Autodesk Inventor part; units mm, degrees
ref_plane "YZ Plane" through (0, 0, 0) normal (1, 0, 0) x (0, 1, 0)
ref_plane "XZ Plane" through (0, 0, 0) normal (0, 1, 0) x (-1, 0, 0)
ref_plane "XY Plane" through (0, 0, 0) normal (0, 0, 1) x (1, 0, 0)
sketch "Szkic1" plane through (0, 0, 0) normal (0, 1, 0) x (-1, 0, 0)
  line L0 (-15, 0) -> (-85, 0)
  line L1 (-100, -15) -> (-100, -100)
  line L2 (-100, -100) -> (0, -100)
  line L3 (0, -100) -> (0, -15)
  arc A0 (0, -15) -> (-15, 0) centre (-15, -15) ccw
  arc A1 (-85, 0) -> (-100, -15) centre (-85, -15) ccw
  point P0 (0, 0)
  point P1 (-100, 0)
  dimension "d0" = 100
  dimension "d1" = 100
  dimension "d2" = 15
extrude "Wyciągnięcie proste1" add sketch "Szkic1" along normal blind 10
sketch "Szkic2" plane through (0, 10, 0) normal (0, 1, 0) x (1, 0, 0)
  line L0 (0, 100) -> (100, 100)
  line L1 (100, 100) -> (100, 50)
  line L2 (100, 50) -> (0, 50)
  line L3 (0, 50) -> (0, 100)
  point P0 (0, 0)
  dimension "d5" = 100
  dimension "d6" = 50
extrude "Wyciągnięcie proste2" add sketch "Szkic2" along normal blind 20
sketch "Szkic3" plane through (0, 10, 0) normal (0, 1, 0) x (1, 0, 0)
  arc A0 (0, 15) -> (15, 0) centre (15, 15) ccw
  arc A1 (85, 0) -> (100, 15) centre (85, 15) ccw
  point P0 (0, 0)
hole "Otwór1" at (15, 10, -15) at (85, 10, -15) direction (0, -1, 0) diameter 16 end through all
mirror "Odbij1" about plane through (50, 30, -75) normal (0, 1, 0) of "Wyciągnięcie proste1", "Otwór1", "Wyciągnięcie proste2"
sketch "Szkic4" plane through (100, 0, -100) normal (0, 0, -1) x (-1, 0, 0)
  circle A0 centre (-40, 19) radius 19
  line L0 (15, 0) -> (0, 0)
  line L1 (0, 0) -> (-40, 0)
  line L2 (-40, 38) -> (0, 38)
  line L3 (0, 10) -> (0, 50)
  line L4 (0, 0) -> (0, 38)
  point P0 (100, 0)
  dimension "d16" = 38
  dimension "d17" = 40
extrude "Wyciągnięcie proste3" add sketch "Szkic4" against normal blind 12
sketch "Szkic5" plane through (100, 60, -100) normal (0, 0, -1) x (-1, 0, 0)
  arc A0 (-40, -22) -> (-40, -60) centre (-40, -41) ccw
  circle A1 centre (-40, -41) radius 19
  point P0 (100, -60)
  point P1 (-40, -22)
  dimension "d20" = 38
extrude "Wyciągnięcie proste4" add sketch "Szkic5" along normal blind 28
sketch "Szkic6" plane through (140, 19, -128) normal (0, 0, -1) x (-1, 0, 0)
  point P0 (140, -19)
  point P1 (0, 0)
hole "Otwór2" at (140, 19, -128) direction (0, 0, 1) diameter 24 end through all
fillet "Zaokrąglenie1" radius 6 1 edges at (100, 19, -88)
sketch "Szkic7" plane through (0, 0, -100) normal (-1, 0, 0) x (0, 0, 1)
  circle A0 centre (19, 100) radius 19
  line L0 (0, 0) -> (0, 60)
  line L1 (0, 60) -> (0, 100)
  line L2 (38, 100) -> (38, 60)
  line L3 (0, 60) -> (85, 60)
  point P0 (100, 0)
  dimension "d31" = 38
  dimension "d32" = 40
extrude "Wyciągnięcie proste5" add sketch "Szkic7" against normal blind 12
sketch "Szkic8" plane through (0, 0, -100) normal (-1, 0, 0) x (0, 0, 1)
  arc A0 (38, 100) -> (0, 100) centre (19, 100) ccw
  circle A1 centre (19, 100) radius 19
  point P0 (100, 0)
  dimension "d35" = 38
extrude "Wyciągnięcie proste6" add sketch "Szkic8" along normal blind 38
sketch "Szkic9" plane through (-38, 100, -81) normal (-1, 0, 0) x (0, 0, 1)
  point P0 (81, -100)
  point P1 (0, 0)
hole "Otwór3" at (-38, 100, -81) direction (1, 0, 0) diameter 22 end through all
fillet "Zaokrąglenie2" radius 6 1 edges at (12, 60, -81)
The listing builds one solid part. Answer for the finished solid, in the listing's coordinates (mm). A direction names the side the tool comes from. Round coordinates to 2 decimals unless told otherwise and drop trailing zeros. Loops run counter-clockwise (first coordinate to the right, second up) from the corner with the lowest first, then second, coordinate; pieces in that order, holes last.
Q1. Section B-B, the plane x = 3 is taken. Determine the outline of the cut face in (y, z).
Q2. Section C-C, the plane z = -26 is taken. Determine the outline of the cut face in (x, y), then the cut area to 3 significant figures.
Q3. Find the intervals of material crossed by line 1 (X direction, y = 6.75, z = -15); line 2 (Z direction, x = 15, y = 7.25); line 3 (Y direction, x = 22, z = -35), in increasing order.
Q4. For a pull along Z with two mould halves and no side action, classify faces 1 (the face through (140.3, 6.6, -128)), 2 (the face through (15, 5, -23)), 3 (the face through (95.72, 4.93, -4.51)) as released by +Z, released by -Z, zero draft, split by the parting line, or undercut.
Q5. Given pin 1 Ø14.5 at (x, y) = (10, 70.5) entering from +Z; pin 2 Ø14.5 at (x, z) = (85, -15) entering from -Y; pin 3 Ø8 at (y, z) = (68, -76.5) entering from +X; pin 4 Ø6 at (x, y) = (116.5, 37.5) entering from -Z, each flat-ended and moving along its own axis, determine where each tip first touches the part or whether it passes through.
Q6. Section A-A, the plane y = 19 is taken. Determine the outline of the cut face in (x, z).
Q7. Section D-D, the plane z = -94.5 is taken. Determine the outline of the cut face in (x, y), then the cut area to 3 significant figures.
Q8. Which of the six approach directions +Z, -Z, +X, -X, +Y, -Y give full straight-line access (tool end or side, diameter ignored) to faces 4 (the face through (127, 19, -88)), 5 (the face through (49, 60, -49)), 6 (the face through (120, 38, -93)), 7 (the face through (-12.65, 118.548, -85.119))?
Completed:
1. outline: (0, -100) - (100, -100) arc R19 ccw to (100, -62) - (60, -62) - (60, -6) - (50, -6) - (50, -50) - (10, -50) - (10, -6) - (0, -6) - close; hole circle Ø22 at (100, -81)
2. outline: (0, 0) - (100, 0) - (100, 10) - (0, 10) - close; (0, 50) - (100, 50) - (100, 60) - (0, 60) - close
2. area: 2,000 mm2
3. line 1: x = 0 to 7, 23 to 77, 93 to 100
3. line 2: z = -100 to -23, -7 to 0
3. line 3: y = 0 to 10, 50 to 60
4. face 1: released by -Z
4. face 2: undercut
4. face 3: released by +Z
5. pin 1: stops at z = -62
5. pin 2: passes through
5. pin 3: stops at x = 12.34
5. pin 4: stops at z = -100
6. outline: (0, -100) - (121, -100) - (121, -128) - (128, -128) - (128, -88) - (106, -88) arc R6 cw to (100, -82) - (100, -50) - (0, -50) - close; (152, -128) - (159, -128) - (159, -88) - (152, -88) - close
7. outline: (-38, 86.63) - (0, 86.63) - (0, 0) - (140, 0) arc R19 ccw to (140, 38) - (100, 38) - (100, 60) - (18, 60) arc R6 cw to (12, 66) - (12, 113.37) - (-38, 113.37) - close; hole circle Ø24 at (140, 19)
7. area: 9,300 mm2
8. face 4: +Z, +X, +Y, -Y
8. face 5: +Z, +X, +Y
8. face 6: +Z, -Z, +X, +Y
8. face 7: -X
